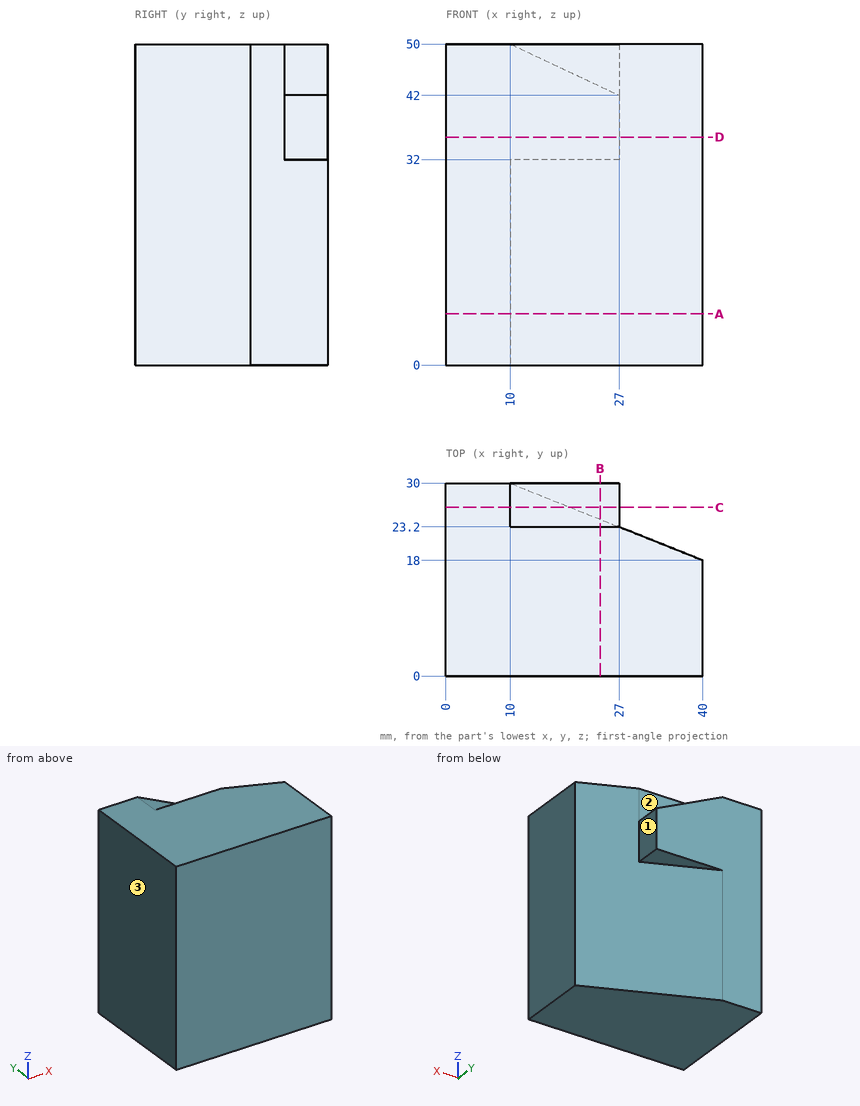
Design review of the part shown in the three views and the two pictorial views. Dimensions are in mm from the part's minimum x, y and z. A direction names the side the tool comes from. Round coordinates to 2 decimals unless told otherwise and drop trailing zeros. Loops run counter-clockwise (first coordinate to the right, second up) from the corner with the lowest first, then second, coordinate; pieces in that order, holes last.
Q1. Add section A-A on z = 8. Write out the cut boundary in (x, y), plus the area to 3 significant figures.
Result sheet:
outline: (0, 0) - (40, 0) - (40, 18) - (10, 30) - (0, 30) - close
area: 1,020 mm2
Q2. Insertion check: pin 1 Ø5.5 at (y, z) = (26, 38) entering from +X; pin 2 Ø6 at (x, z) = (27, 20) entering from +Y. Each pin has a flat end and moves straight along its axis. Give the tip position at first contact, or say it passes through.
Result sheet:
pin 1: stops at x = 27
pin 2: stops at y = 24.4
Q3. Add section C-C on y = 26.25. Write out the cut boundary in (x, z) (3 decimals).
Result sheet:
outline: (0, 0) - (19.375, 0) - (19.375, 32) - (27, 32) - (27, 42) - (10, 50) - (0, 50) - close
Q4. Machinability: for the marked faces 1, 2 and 3, which of the approach directions +Z, -Z, +X, -X, +Y, -Y give a long, thin tool a straight path to every point of the face, cutting with its end or side? Answer none if there is none.
Result sheet:
face 1: +Z, -Z, +X, +Y
face 2: +Z, +X, +Y
face 3: +Z, -Z, -X, +Y, -Y
Q5. Add section B-B on x = 24. Write out the cut boundary in (y, z), plus the area to 3 significant figures.
Result sheet:
outline: (0, 0) - (24.4, 0) - (24.4, 32) - (30, 32) - (30, 43.41) - (23.2, 43.41) - (23.2, 50) - (0, 50) - close
area: 1,280 mm2
Q6. To check wall thickness, follow line 1 along Y through (x, z) = (27, 13); line 2 along X through (y, z) = (28.75, 37); line 3 along Z through (x, y) = (24, 23.5). State the ranges of each line that lie inside material, in increasing order.
Result sheet:
line 1: y = 0 to 23.2
line 2: x = 0 to 27
line 3: z = 0 to 43.41
Q7. Add section D-D on z = 35.5. Write out the cut boundary in (x, y).
Result sheet:
outline: (0, 0) - (40, 0) - (40, 18) - (27, 23.2) - (27, 30) - (0, 30) - close
